For this review, take the finished solid that the model builds, in its own axes (mm). A direction names the side the tool comes from. Give positions to 0.01 mm unless a question says otherwise; leave off trailing zeros. Loops run counter-clockwise (first coordinate to the right, second up) from the corner with the lowest first, then second, coordinate; pieces in that order, holes last. Notation, with made-up numbers: (45, 51) - (81, 51) arc R32 ccw to (81, 77) - close; hole circle Ø10 at (-3.75, -9.75). An arc over 180 degrees is marked (long way). Answer in a Markdown table with one row per item.
```python
from build123d import *

# Parameters (mm, degrees)
F1_DEPTH = 600
F2_W     = 5
F2_H     = 80
F3_DEPTH = 25
F4_R     = 2
F5_W     = 4.5
F5_H     = 80
F6_DEPTH = 132.001
F7_R     = 2
F9_DEPTH = 7.5


with BuildPart() as f1:
    # F0 (on Top) → F1 (new body)
    with BuildSketch(Plane.XY):
        with BuildLine():
            Line((-60, 0), (-66, 0))
            Line((-66, 0), (-66, -51))
            ThreePointArc((-66, -51), (-61.606602, -61.606602), (-51, -66))
            Line((-51, -66), (51, -66))
            ThreePointArc((51, -66), (61.606602, -61.606602), (66, -51))
            Line((66, -51), (66, 0))
            Line((66, 0), (60, 0))
            Line((60, 0), (60, -51))
            ThreePointArc((60, -51), (57.363961, -57.363961), (51, -60))
            Line((51, -60), (-51, -60))
            ThreePointArc((-51, -60), (-57.363961, -57.363961), (-60, -51))
            Line((-60, -51), (-60, 0))
        make_face()
    extrude(amount=F1_DEPTH)

    # F2 (on face) → F3 (cut)
    with BuildSketch(Plane.XZ.offset(66)):
        with Locations((-43.75, 525)):
            Rectangle(F2_W, F2_H)
        with Locations((-31.25, 525)):
            Rectangle(F2_W, F2_H)
        with Locations((-18.75, 525)):
            Rectangle(F2_W, F2_H)
        with Locations((-6.25, 525)):
            Rectangle(F2_W, F2_H)
        with Locations((6.25, 525)):
            Rectangle(F2_W, F2_H)
        with Locations((18.75, 525)):
            Rectangle(F2_W, F2_H)
        with Locations((31.25, 525)):
            Rectangle(F2_W, F2_H)
        with Locations((43.75, 525)):
            Rectangle(F2_W, F2_H)
    extrude(amount=-F3_DEPTH, mode=Mode.SUBTRACT)

    # F4
    f4_edges = [f1.edges().sort_by_distance(p)[0] for p in [
        (-46.25, -63, 485),
        (-33.75, -63, 485),
        (-21.25, -63, 485),
        (-8.75, -63, 485),
        (3.75, -63, 485),
        (16.25, -63, 485),
        (28.75, -63, 485),
        (41.25, -63, 485),
        (-46.25, -63, 565),
        (-33.75, -63, 565),
        (-21.25, -63, 565),
        (-8.75, -63, 565),
        (3.75, -63, 565),
        (16.25, -63, 565),
        (28.75, -63, 565),
        (41.25, -63, 565),
        (-41.25, -63, 565),
        (-28.75, -63, 565),
        (-16.25, -63, 565),
        (-3.75, -63, 565),
        (8.75, -63, 565),
        (21.25, -63, 565),
        (33.75, -63, 565),
        (46.25, -63, 565),
        (46.25, -63, 485),
        (33.75, -63, 485),
        (21.25, -63, 485),
        (8.75, -63, 485),
        (-3.75, -63, 485),
        (-16.25, -63, 485),
        (-28.75, -63, 485),
        (-41.25, -63, 485),
    ]]
    fillet(f4_edges, radius=F4_R)

    # F5 (on face) → F6 (cut, through all)
    with BuildSketch(Plane.YZ.offset(66)):
        with Locations((-42, 525)):
            Rectangle(F5_W, F5_H)
        with Locations((-30, 525)):
            Rectangle(F5_W, F5_H)
        with Locations((-18, 525)):
            Rectangle(F5_W, F5_H)
        with Locations((-6, 525)):
            Rectangle(F5_W, F5_H)
    extrude(amount=-F6_DEPTH, mode=Mode.SUBTRACT)

    # F7
    f7_edges = [f1.edges().sort_by_distance(p)[0] for p in [
        (-63, -3.75, 485),
        (63, -3.75, 485),
        (-63, -15.75, 485),
        (63, -15.75, 485),
        (-63, -27.75, 485),
        (63, -27.75, 485),
        (-63, -39.75, 485),
        (63, -39.75, 485),
        (-63, -44.25, 485),
        (63, -44.25, 485),
        (-63, -32.25, 485),
        (63, -32.25, 485),
        (-63, -20.25, 485),
        (63, -20.25, 485),
        (-63, -8.25, 485),
        (63, -8.25, 485),
        (-63, -39.75, 565),
        (63, -39.75, 565),
        (-63, -27.75, 565),
        (63, -27.75, 565),
        (-63, -15.75, 565),
        (63, -15.75, 565),
        (-63, -3.75, 565),
        (63, -3.75, 565),
        (-63, -8.25, 565),
        (63, -8.25, 565),
        (-63, -20.25, 565),
        (63, -20.25, 565),
        (-63, -32.25, 565),
        (63, -32.25, 565),
        (-63, -44.25, 565),
        (63, -44.25, 565),
    ]]
    fillet(f7_edges, radius=F7_R)

    # F8 (on face) → F9 (cut)
    with BuildSketch(Plane.XY.offset(600)):
        with BuildLine():
            Line((-63, -51), (-63, 0))
            Line((-63, 0), (-66, 0))
            Line((-66, 0), (-66, -51))
            ThreePointArc((-66, -51), (-61.606602, -61.606602), (-51, -66))
            Line((-51, -66), (51, -66))
            ThreePointArc((51, -66), (61.606602, -61.606602), (66, -51))
            Line((66, -51), (66, 0))
            Line((66, 0), (63, 0))
            Line((63, 0), (63, -51))
            ThreePointArc((63, -51), (59.485281, -59.485281), (51, -63))
            Line((51, -63), (-51, -63))
            ThreePointArc((-51, -63), (-59.485281, -59.485281), (-63, -51))
        make_face()
    extrude(amount=-F9_DEPTH, mode=Mode.SUBTRACT)


solid = f1.part
```
1. We need section A-A, the plane z = 354. Give the boundary of the cut face in (x, y).
Values:
| item | result |
|---|---|
| outline | (-66, -51) arc R15 ccw to (-51, -66) - (51, -66) arc R15 ccw to (66, -51) - (66, 0) - (60, 0) - (60, -51) arc R9 cw to (51, -60) - (-51, -60) arc R9 cw to (-60, -51) - (-60, 0) - (-66, 0) - close |
2. We need section B-B, the plane z = 538. Count the separate pieces of the cut face and the enclosed holes in it, and give its area (3 significant figures).
Values:
| item | result |
|---|---|
| separate pieces | 17 |
| enclosed holes | 0 |
| area | 994 mm^2 |
3. Wall thickness on line 1 (X direction, y = -11, z = 56.5); line 2 (Y direction, x = 7, z = 270); line 3 (X direction, y = -53.5, z = 459.5): over which ranges is each line inside the solid? List them lowest first. Write a range as [from, to].
Values:
| item | result |
|---|---|
| line 1 | x = [-66, -60], [60, 66] |
| line 2 | y = [-66, -60] |
| line 3 | x = [-65.79, -59.65], [59.65, 65.79] |
4. Clearance check with flat-ended pins moving along their axes: pin 1 (1.8 mm diameter, centred on y = -64, z = 538.5, fed in from -X); pin 2 (3 mm diameter, centred on x = 64.5, z = 516.5, fed in from -Y); pin 3 (6.5 mm diameter, centred on y = -62.5, z = 526, fed in from +X); pin 4 (3 mm diameter, centred on x = -63.5, z = 540, fed in from +Y). State where each tip first meets the part, or that it passes through.
Values:
| item | result |
|---|---|
| pin 1 | stops at x = -59.87 |
| pin 2 | stops at y = -60 |
| pin 3 | stops at x = 63.53 |
| pin 4 | stops at y = 0 |
5. Mouldability with a two-part tool opening along X and no side actions: class faces 1 (the face through (-59.39, -59.58, 596.3)), 2 (the face through (0, -62, 0)), 3 (the face through (1, -60, 296)) as released by +X, released by -X, zero draft, split by the parting line, or undercut.
Values:
| item | result |
|---|---|
| face 1 | released by -X |
| face 2 | zero draft |
| face 3 | undercut |
6. For faces 4 (the face through (66, -26, 292)), 5 (the face through (0, -65, 592.5)), 6 (the face through (60, -25, 296)), 7 (the face through (59.58, -59.39, 596.3)), list the 3-axis set-ups (+Z, -Z, +X, -X, +Y, -Y) from which the entire face can be reached by the end or side of a thin tool; tool diameter is ignored.
Values:
| item | result |
|---|---|
| face 4 | +Z, -Z, +X, +Y, -Y |
| face 5 | +Z, -Y |
| face 6 | +Z, -Z, +Y |
| face 7 | +Z, +X, -Y |
